Autodesk Inventor part; units mm, degrees
ref_plane "YZ Plane" through (0, 0, 0) normal (1, 0, 0) x (0, 1, 0)
ref_plane "XZ Plane" through (0, 0, 0) normal (0, 1, 0) x (-1, 0, 0)
ref_plane "XY Plane" through (0, 0, 0) normal (0, 0, 1) x (1, 0, 0)
sketch "Sketch1" plane through (0, 0, 0) normal (0, 0, 1) x (1, 0, 0)
  circle A0 centre (0, 0) radius 1.5
  arc A1 (-8.6933, 2.3294) -> (0, 9) centre (0, 0) ccw
  line L0 (0, 2) -> (0, 9)
  line L1 (-1.9319, 0.5176) -> (-8.6933, 2.3294)
  arc A2 (0, 2) -> (-1.9319, 0.5176) centre (0, 0) ccw
extrude "Extrusion1" add sketch "Sketch1" along normal blind 3.6
sketch "Sketch2" plane through (0, 0, 3.6) normal (0, 0, 1) x (1, 0, 0)
  circle A0 centre (4.1719, 4.1719) radius 2.1
extrude "Extrusion2" cut sketch "Sketch2" against normal blind 3
properties part number "cam"
Model file for the job. Use its own axes, mm. A direction names the side the tool comes from. Coordinates: 2 decimals unless noted, no trailing zeros. Write each loop counter-clockwise with the first axis right and the second up, starting at its lowest first coordinate (ties: lowest second). Pieces come first, ordered by that corner, then holes. Notation, with made-up numbers: (18, 42.25) - (52, 42.25) arc R22 ccw to (52, 51.25) - close; hole circle Ø7 at (46, -18). An arc over 180 degrees is marked (long way). One line per item, written item: value. Start each with the question number.
1. Mould opens along Y. For faces 1 (the flat face through (0, -2, 3.6)), 2 (the cylindrical face through (5.301, 5.943, 2.121)), 3 (the cylindrical face through (5.72, -6.95, 1.77)) say: released by +Y, released by -Y, zero draft, split by the parting line, or undercut.
2. Slice it at C-C (z = 2.45). Write the cut outline in (x, y).
3. Slice it at A-A (y = 0). Write the cut outline in (x, z).
4. Slice it at D-D (x = 3). Write the cut outline in (y, z), plus the area to 3 significant figures.
5. Flat gauge pins, fed straight in: pin 1 (2 mm diameter, centred on x = 4, y = 4, fed in from +Z); pin 2 (3.5 mm diameter, centred on x = 4.17, y = 4.17, fed in from -Z); pin 3 (1.8 mm diameter, centred on x = 0, y = 0, fed in from +Z). Where does each tip first touch, or does it go through?
6. Slice it at B-B (x = -0.5). Write the cut outline in (y, z), plus the area to 3 significant figures.
7. Tool access for faces 4 (the cylindrical face through (-1.2, 1.6, 1.8)), 5 (the cylindrical face through (-1.5, -0.07, 1.77)), 6 (the flat face through (4, 4, 0.6)): list every direction of +Z, -Z, +X, -X, +Y, -Y with a clear straight run to the whole face (end or side of a thin tool).
8. Probe line 1 (X direction, y = 8.25, z = 1.9); line 2 (Y direction, x = 2.5, z = 1.9); line 3 (X direction, y = 3.5, z = 2.1). List the from-to ranges inside material, lowest first. Write a range as from..to.
Answers below:
1. face 1: zero draft
1. face 2: undercut
1. face 3: split by the parting line
2. outline: (-8.69, 2.33) arc R9 ccw (long way) to (0, 9) - (0, 2) arc R2 ccw to (-1.93, 0.52) - close; hole circle Ø3 at (0, 0); hole circle Ø4.2 at (4.17, 4.17)
3. outline: (-9, 0) - (-1.5, 0) - (-1.5, 3.6) - (-9, 3.6) - close; (1.5, 0) - (9, 0) - (9, 3.6) - (1.5, 3.6) - close
4. outline: (-8.49, 0) - (8.49, 0) - (8.49, 3.6) - (5.91, 3.6) - (5.91, 0.6) - (2.43, 0.6) - (2.43, 3.6) - (-8.49, 3.6) - close
4. area: 50.6 mm^2
5. pin 1: stops at z = 0.6
5. pin 2: stops at z = 0
5. pin 3: passes through
6. outline: (-8.99, 0) - (-1.41, 0) - (-1.41, 3.6) - (-8.99, 3.6) - close; (1.41, 0) - (1.94, 0) - (1.94, 3.6) - (1.41, 3.6) - close
6. area: 29.1 mm^2
7. face 4: +Z, -Z, +Y
7. face 5: +Z, -Z
7. face 6: +Z
8. line 1: x = 0..3.6
8. line 2: y = -8.65..2.9, 5.44..8.65
8. line 3: x = 0..2.18, 6.16..8.29
